Part model, mm, in its own coordinate system. Face numbers are marked on the shaded views. A direction names the side the tool comes from. Round coordinates to 2 decimals unless told otherwise and drop trailing zeros. Write each loop counter-clockwise with the first axis right and the second up, starting at its lowest first coordinate (ties: lowest second). Pieces come first, ordered by that corner, then holes. Notation, with made-up numbers: (1.5, 85.5) -> (56.5, 85.5) arc R17 ccw to (56.5, 107.5) -> close; hole circle Ø11 at (55, -19). An arc over 180 degrees is marked (long way). Return JSON: item names as keys, results as strings. Group by question number.
(1) Saw through at A-A (x = 0). List the corners of the cut face in (y, z), plus the area to 3 significant figures.
(2) Drop flat-ended pins along their axis: pin 1 Ø21 at (x, z) = (10.5, -71.5) entering from +Y; pin 2 Ø21 at (x, y) = (1, -110.5) entering from +Z; pin 3 Ø8 at (x, z) = (14.5, -229) entering from +Y. Give the stop position or say it passes through.
(3) Drill centre lines: L1, parallel to Z at x = 0, y = -117; L2, parallel to Z at x = 19, y = -63.5; L3, parallel to Y at x = 0, z = 22. Where is each one in solid material? Low to high. Write a range as from..to.
(4) Mould opens along Y. For the marked faces 1, 2, 3 and 4 say: +Y half, -Y half, draft (parallel to the pull), parting line (faces both ways), or undercut.
(5) Saw through at C-C (z = 14). List the corners of the cut face in (x, y).
(6) Saw through at B-B (y = -78). List the corners of the cut face in (x, z).
(7) Saw through at D-D (x = 16). List the corners of the cut face in (y, z).
(8) Tool access for the marked faces 5, 6 and 7: list every direction of +Z, -Z, +X, -X, +Y, -Y with a clear straight run to the whole face (end or side of a thin tool).
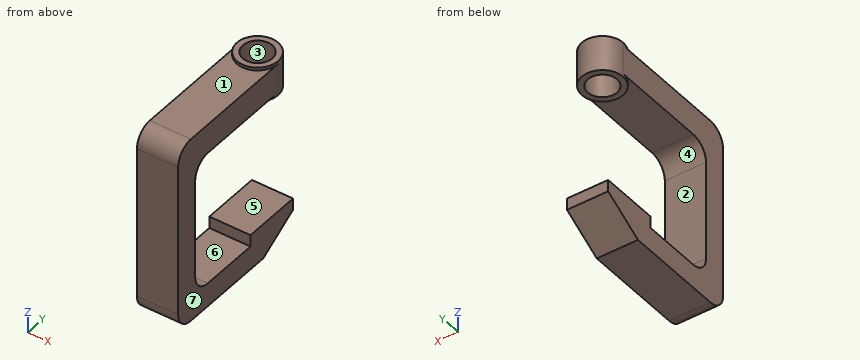
Autodesk Inventor part; units mm, degrees
ref_plane "YZ Plane" through (0, 0, 0) normal (1, 0, 0) x (0, 1, 0)
ref_plane "XZ Plane" through (0, 0, 0) normal (0, 1, 0) x (-1, 0, 0)
ref_plane "XY Plane" through (0, 0, 0) normal (0, 0, 1) x (1, 0, 0)
sketch "Esboço1" plane through (0, 0, 0) normal (0, 0, 1) x (1, 0, 0)
  circle A0 centre (0, 0) radius 25
  circle A1 centre (0, 0) radius 35
  dimension "d0" = 50
  dimension "d1" = 70
extrude "Extrusão1" add sketch "Esboço1" along normal blind 60
sketch "Esboço2" plane through (0, 0, 0) normal (1, 0, 0) x (0, 1, 0)
  line L0 (35, 0) -> (-35, 0) construction
  line L1 (-35, 0) -> (-35, 5) construction
  line L2 (-35, 0) -> (-35, 60) construction
  line L3 (-35, 5) -> (-195, 5)
  line L4 (-35, 60) -> (-35, 55) construction
  line L5 (-35, 55) -> (-235, 55)
  line L6 (-235, 55) -> (-235, -265)
  line L7 (-235, -265) -> (-35, -265)
  line L8 (-35, -265) -> (35, -224.5855)
  line L9 (35, 0) -> (35, -224.5855) construction
  line L10 (35, -224.5855) -> (35, -204.5855)
  line L11 (35, -204.5855) -> (-65, -204.5855)
  line L12 (-65, -204.5855) -> (-65, -224.5855)
  line L13 (-65, -224.5855) -> (-195, -224.5855)
  line L14 (-195, -224.5855) -> (-195, 5)
  line L15 (-35, 55) -> (-35, 5)
  point P0 (0, 0)
  dimension "d4" = 5
  dimension "d5" = 160
  dimension "d6" = 5
  dimension "d7" = 200
  dimension "d8" = 320
  dimension "d9" = 200
  dimension "d10" = 150
  dimension "d11" = 20
  dimension "d12" = 100
  dimension "d13" = 20
  dimension "d14" = 130
extrude "Extrusão2" add sketch "Esboço2" along normal mid plane 70
fillet "Arredondamento1" radius 30 4 edges at (0, -235, 55) (0, -195, 5) (0, -235, -265) (0, -195, -224.5855)
sketch "Esboço3" plane through (-35, -35, 5) normal (0, 1, 0) x (1, 0, 0)
  line L0 (70, -20) -> (70, -50)
  line L1 (0, 0) -> (70, 0)
  line L2 (70, -50) -> (0, -50)
  line L3 (0, -50) -> (0, 0)
  line L4 (0, 0) -> (70, 0)
  line L5 (70, 0) -> (70, -50)
  point P0 (35, 5)
extrude "Extrusão3" add sketch "Esboço3" along normal up to next
thread "Rosca1"
properties part number "Corpo da Morsa"
Computed values:
{
 "1": {"outline": "(-235, -235) arc R30 ccw to (-205, -265) -> (-35, -265) -> (35, -224.59) -> (35, -204.59) -> (-65, -204.59) -> (-65, -224.59) -> (-165, -224.59) arc R30 cw to (-195, -194.59) -> (-195, -25) arc R30 cw to (-165, 5) -> (-35, 5) -> (-35, 0) -> (-25, 0) -> (-25, 60) -> (-35, 60) -> (-35, 55) -> (-205, 55) arc R30 ccw to (-235, 25) -> close; (25, 0) -> (35, 0) -> (35, 60) -> (25, 60) -> close", "area": "31,900 mm2"},
 "2": {"pin 1": "y = -195", "pin 2": "z = 55", "pin 3": "y = 34.28"},
 "3": {"L1": "-265..-224.59, 5..55", "L2": "-265..-204.59, 5..55", "L3": "-235..-25, 25..35"},
 "4": {"face 1": "draft", "face 2": "+Y half", "face 3": "undercut", "face 4": "undercut"},
 "5": {"outline": "(-35, -235) -> (35, -235) -> (35, 0) arc R35 ccw to (-35, 0) -> close; hole circle Ø50 at (0, 0)"},
 "6": {"outline": "(-35, -265) -> (35, -265) -> (35, -224.59) -> (-35, -224.59) -> close; (-35, 5) -> (35, 5) -> (35, 55) -> (-35, 55) -> close"},
 "7": {"outline": "(-235, -235) arc R30 ccw to (-205, -265) -> (-35, -265) -> (35, -224.59) -> (35, -204.59) -> (-65, -204.59) -> (-65, -224.59) -> (-165, -224.59) arc R30 cw to (-195, -194.59) -> (-195, -25) arc R30 cw to (-165, 5) -> (-31.13, 5) -> (-31.13, 0) -> (-19.21, 0) -> (-19.21, 60) -> (-31.13, 60) -> (-31.13, 55) -> (-205, 55) arc R30 ccw to (-235, 25) -> close; (19.21, 0) -> (31.13, 0) -> (31.13, 60) -> (19.21, 60) -> close"},
 "8": {"face 5": "+X, -X, +Y", "face 6": "+X, -X", "face 7": "+Z, -Z, +X, +Y, -Y"}
}
